Work out the finished part from the listing and answer in its coordinate system (mm). A direction names the side the tool comes from. Give positions to 0.01 mm unless a question says otherwise; leave off trailing zeros. Order: outer loops, then holes, each group sorted by start corner. A loop starts at its lowest first (then second) coordinate and runs counter-clockwise, first axis right, second up. Notation, with made-up numbers: (-37.5, -26) - (-14.5, -26) arc R12 cw to (-14.5, -17) - close; hole circle Ø8 at (31, 84.25). An arc over 180 degrees is marked (long way). Write each question's results on one line, items separated by ' | '.
from build123d import *

# Parameters (mm, degrees)
BOSS_EXTRUDE3_DEPTH = 25.4
CUT_EXTRUDE4_REACH  = 182.233
SKETCH2_W           = 19.05
SKETCH2_H           = 19.05
CUT_EXTRUDE5_DEPTH  = 25.4
SKETCH4_R           = 3.988266949
CUT_EXTRUDE6_DEPTH  = 3.175
SKETCH5_R           = 3.175
CUT_EXTRUDE7_DEPTH  = 3.175


with BuildPart() as part:
    # Sketch1 → Boss-Extrude3 (new body)
    with BuildSketch(Plane(origin=(0, 0, 0), x_dir=(1, 0, 0), z_dir=(0, 1, 0))):
        Polygon((73.659861316, 0), (108.190600856, 0), (0, 117.475), (-18.683642708, 100.267981224), align=None)
    extrude(amount=BOSS_EXTRUDE3_DEPTH)

    # Cut-Extrude4: up to this plane
    cut_extrude4_end = Plane(origin=(0, 25.4, 0), z_dir=(0, 0, -1))
    # Sketch2 → Cut-Extrude4 (cut, up to the surface)
    with BuildSketch(Plane(origin=(-58.537665842, 0, -63.563740241), x_dir=(0.735576484560878, 0, -0.6774416841035549), z_dir=(0.6774416841035549, 0, 0.735576484560878)), mode=Mode.PRIVATE) as cut_extrude4_sk1:
        with Locations((66.880665058, 12.7)):
            Rectangle(SKETCH2_W, SKETCH2_H)
    cut_extrude4_tool1 = split(extrude(cut_extrude4_sk1.sketch, amount=CUT_EXTRUDE4_REACH, mode=Mode.PRIVATE), bisect_by=cut_extrude4_end, keep=Keep.BOTH, mode=Mode.PRIVATE)
    add(cut_extrude4_tool1.solids().sort_by_distance((-9.341821, 12.7, -108.871491))[0], mode=Mode.SUBTRACT)

    # Sketch3 → Cut-Extrude5 (cut)
    with BuildSketch(Plane(origin=(0, 25.4, 0), x_dir=(1, 0, 0), z_dir=(0, 1, 0))):
        Polygon((0, 117.475), (0, 79.980997791), (-18.683642708, 100.267981224), align=None)
        Polygon((108.190600856, 0), (73.659861316, 0), (89.250643344, -17.183967795), align=None)
    extrude(amount=-CUT_EXTRUDE5_DEPTH, mode=Mode.SUBTRACT)

    # Sketch4 → Cut-Extrude6 (cut)
    with BuildSketch(Plane(origin=(0, 25.4, 0), x_dir=(1, 0, 0), z_dir=(0, 1, 0))):
        with Locations(Location((83.819861316, 12.7, 0), (0, 0, 270))):
            Circle(SKETCH4_R)
    cut_extrude6 = extrude(amount=-CUT_EXTRUDE6_DEPTH, mode=Mode.SUBTRACT)

    # Mirror1: Cut-Extrude6 across plane
    add(cut_extrude6.mirror(Plane.ZX.offset(12.7)), mode=Mode.SUBTRACT)

    # Sketch5 → Cut-Extrude7 (cut)
    with BuildSketch(Plane.XZ):
        with Locations(Location((12.7, -89.535, 0), (0, 0, 270))):
            Circle(SKETCH5_R)
    cut_extrude7 = extrude(amount=-CUT_EXTRUDE7_DEPTH, mode=Mode.SUBTRACT)

    # Mirror2: Cut-Extrude7 across plane
    add(cut_extrude7.mirror(Plane.ZX.offset(12.7)), mode=Mode.SUBTRACT)


solid = part.part
1. A tool of negligible diameter and unlimited length cuts with its end or side. For faces 1 (the face through (44, 22.225, -51)), 2 (the face through (91, 24, 0)), from which of +Z, -Z, +X, -X, +Y, -Y can it reach the whole face along a straight path? Write none if from no direction.
Answer list:
face 1: none | face 2: +Z, +X, -X, +Y, -Y
2. A cutting plane is placed at C-C, the plane y = 15.75. Write down the section's boundary in (x, z) (3 decimals).
Answer list:
outline: (0, -117.475) - (108.191, 0) - (103.874, 0) - (0, -112.788) - close; (0, -84.668) - (77.976, 0) - (73.66, 0) - (0, -79.981) - close
3. Determine the mould class of faces 3 (the face through (0, 2, -99)), 4 (the face through (44, 3.175, -51)), 5 (the face through (54.85, 12.52, -57.92)) for opening direction X: +X half, -X half, draft (parallel to the pull), parting line (faces both ways), or undercut.
Answer list:
face 3: -X half | face 4: undercut | face 5: +X half
4. A cutting plane is placed at D-D, the plane x = 71.5. Write down the section's boundary in (y, z) (3 decimals), then the cut area to 3 significant figures.
Answer list:
outline: (0, -39.839) - (25.4, -39.839) - (25.4, -2.345) - (0, -2.345) - close; hole (3.175, -35.152) - (22.225, -35.152) - (22.225, -7.032) - (3.175, -7.032) - close | area: 417 mm^2
5. A cutting plane is placed at B-B, the plane x = 12.7. Write down the section's boundary in (y, z) (3 decimals).
Answer list:
outline: (0, -103.685) - (25.4, -103.685) - (25.4, -92.71) - (22.225, -92.71) - (22.225, -98.998) - (3.175, -98.998) - (3.175, -92.71) - (0, -92.71) - close; (0, -86.36) - (3.175, -86.36) - (3.175, -70.878) - (22.225, -70.878) - (22.225, -86.36) - (25.4, -86.36) - (25.4, -66.191) - (0, -66.191) - close
6. A cutting plane is placed at A-A, the plane z = -12.7. Write down the section's boundary in (x, y) (3 decimals).
Answer list:
outline: (61.964, 0) - (79.832, 0) - (79.832, 3.175) - (66.28, 3.175) - (66.28, 22.225) - (79.832, 22.225) - (79.832, 25.4) - (61.964, 25.4) - close; (87.808, 0) - (96.494, 0) - (96.494, 25.4) - (87.808, 25.4) - (87.808, 22.225) - (92.178, 22.225) - (92.178, 3.175) - (87.808, 3.175) - close
7. Given P1, Ø3, axis at y = 3, z = -24.5, coming from the -X side; P2, Ø8, axis at y = 19, z = -47.5, coming from the +X side; P3, Ø6, axis at x = 68.5, y = 15, coming from the +Z side, each flat-ended and moving along its own axis, determine where each tip first touches the part or whether it passes through.
Answer list:
P1: x = 49.71 | P2: x = 68.13 | P3: z = -2.35
8. Straight lines are drawn through the part: line 1 (Y direction, x = 61, z = -19.5) (3 decimals); line 2 (X direction, y = 21, z = -28.5); line 3 (X direction, y = 18, z = -40.5). For each, find the intervals that lie inside material, in ascending order. Write a range as [from, to].
Answer list:
line 1: [0, 3.175], [22.225, 25.4] | line 2: [47.41, 51.73], [77.63, 81.94] | line 3: [36.36, 40.68], [66.58, 70.89]
